Input: part model. Units: mm. Frame: model coordinates. Round coordinates to 2 decimals unless told otherwise and drop trailing zeros. Loops run counter-clockwise (first coordinate to the right, second up) from the corner with the lowest first, then second, coordinate; pieces in that order, holes last. Notation, with made-up numbers: (10.5, -22.5) -> (36.5, -22.5) arc R27 cw to (36.5, 2.5) -> close; hole circle Ø6 at (-36, 30). An arc over 180 degrees is marked (long way). One line per question, with ' | ' between items. Start each with the question number.
Q1. Cut plane C-C on y = 31.5. Return loops of the section in (x, z) (3 decimals).
Q2. Cut plane B-B on x = 1.95. State how many separate pieces and enclosed holes the cut face has, and give its area (3 significant figures).
Q3. Material intervals for L1, parallel to Z at x = 1.9, y = 4; L2, parallel to Y at x = 0.65, z = -15; L3, parallel to Y at x = 0.2, z = -73, sorted ascending.
Q4. Cut plane D-D on z = -70.5. Return loops of the section in (x, y) (3 decimals).
Q5. Cut plane A-A on z = -8. Return loops of the section in (x, y) (3 decimals).
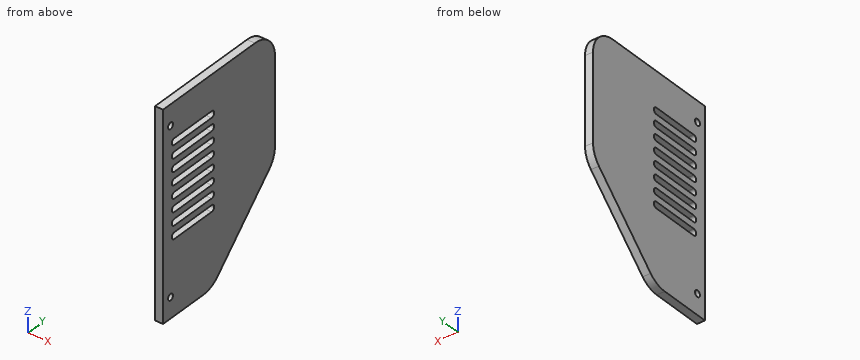
from build123d import *

# Parameters (mm, degrees)
SKETCH1_R           = 1.27
BOSS_EXTRUDE1_DEPTH = 3.175
FILLET1_R           = 10.16


with BuildPart() as part:
    # Sketch1 → Boss-Extrude1 (new body)
    with BuildSketch(Plane(origin=(0, 0, 0), x_dir=(0, 0, -1), z_dir=(1, 0, 0))):
        Polygon((0, 0), (81.026, 0), (81.026, 24.694077964), (48.697077964, 57.023), (0, 57.023), align=None)
        with Locations((8.128, 3.81)):
            Circle(SKETCH1_R, mode=Mode.SUBTRACT)
        with Locations((72.898, 3.81)):
            Circle(SKETCH1_R, mode=Mode.SUBTRACT)
        with BuildLine():
            Line((51.943, 24.765), (51.943, 5.715))
            ThreePointArc((51.943, 5.715), (50.673, 4.445), (49.403, 5.715))
            Line((49.403, 5.715), (49.403, 24.765))
            ThreePointArc((49.403, 24.765), (50.673, 26.035), (51.943, 24.765))
        make_face(mode=Mode.SUBTRACT)
        with BuildLine():
            Line((46.863, 24.765), (46.863, 5.715))
            ThreePointArc((46.863, 5.715), (45.593, 4.445), (44.323, 5.715))
            Line((44.323, 5.715), (44.323, 24.765))
            ThreePointArc((44.323, 24.765), (45.593, 26.035), (46.863, 24.765))
        make_face(mode=Mode.SUBTRACT)
        with BuildLine():
            Line((16.383, 24.765), (16.383, 5.715))
            ThreePointArc((16.383, 5.715), (15.113, 4.445), (13.843, 5.715))
            Line((13.843, 5.715), (13.843, 24.765))
            ThreePointArc((13.843, 24.765), (15.113, 26.035), (16.383, 24.765))
        make_face(mode=Mode.SUBTRACT)
        with BuildLine():
            Line((41.783, 24.765), (41.783, 5.715))
            ThreePointArc((41.783, 5.715), (40.513, 4.445), (39.243, 5.715))
            Line((39.243, 5.715), (39.243, 24.765))
            ThreePointArc((39.243, 24.765), (40.513, 26.035), (41.783, 24.765))
        make_face(mode=Mode.SUBTRACT)
        with BuildLine():
            Line((36.703, 24.765), (36.703, 5.715))
            ThreePointArc((36.703, 5.715), (35.433, 4.445), (34.163, 5.715))
            Line((34.163, 5.715), (34.163, 24.765))
            ThreePointArc((34.163, 24.765), (35.433, 26.035), (36.703, 24.765))
        make_face(mode=Mode.SUBTRACT)
        with BuildLine():
            Line((31.623, 24.765), (31.623, 5.715))
            ThreePointArc((31.623, 5.715), (30.353, 4.445), (29.083, 5.715))
            Line((29.083, 5.715), (29.083, 24.765))
            ThreePointArc((29.083, 24.765), (30.353, 26.035), (31.623, 24.765))
        make_face(mode=Mode.SUBTRACT)
        with BuildLine():
            Line((26.543, 24.765), (26.543, 5.715))
            ThreePointArc((26.543, 5.715), (25.273, 4.445), (24.003, 5.715))
            Line((24.003, 5.715), (24.003, 24.765))
            ThreePointArc((24.003, 24.765), (25.273, 26.035), (26.543, 24.765))
        make_face(mode=Mode.SUBTRACT)
        with BuildLine():
            Line((21.463, 24.765), (21.463, 5.715))
            ThreePointArc((21.463, 5.715), (20.193, 4.445), (18.923, 5.715))
            Line((18.923, 5.715), (18.923, 24.765))
            ThreePointArc((18.923, 24.765), (20.193, 26.035), (21.463, 24.765))
        make_face(mode=Mode.SUBTRACT)
    extrude(amount=BOSS_EXTRUDE1_DEPTH)

    # Fillet1
    fillet1_edges = [part.edges().sort_by_distance(p)[0] for p in [
        (1.5875, 57.023, -48.697077964),
        (1.5875, 24.694077964, -81.026),
        (1.5875, 57.023, 0),
    ]]
    fillet(fillet1_edges, radius=FILLET1_R)


solid = part.part
Results:
1) outline: (0, -74.22) -> (3.175, -74.22) -> (3.175, 0) -> (0, 0) -> close
2) separate pieces: 1 | enclosed holes: 10 | area: 3,630 mm^2
3) L1: -81.03 to -74.15, -71.64 to -9.38, -6.87 to 0 | L2: 0 to 4.45, 26.03 to 57.02 | L3: 0 to 2.54, 5.08 to 32.72
4) outline: (0, 0) -> (3.175, 0) -> (3.175, 35.22) -> (0, 35.22) -> close
5) outline: (0, 0) -> (3.175, 0) -> (3.175, 2.546) -> (0, 2.546) -> close; (0, 5.074) -> (3.175, 5.074) -> (3.175, 56.791) -> (0, 56.791) -> close
